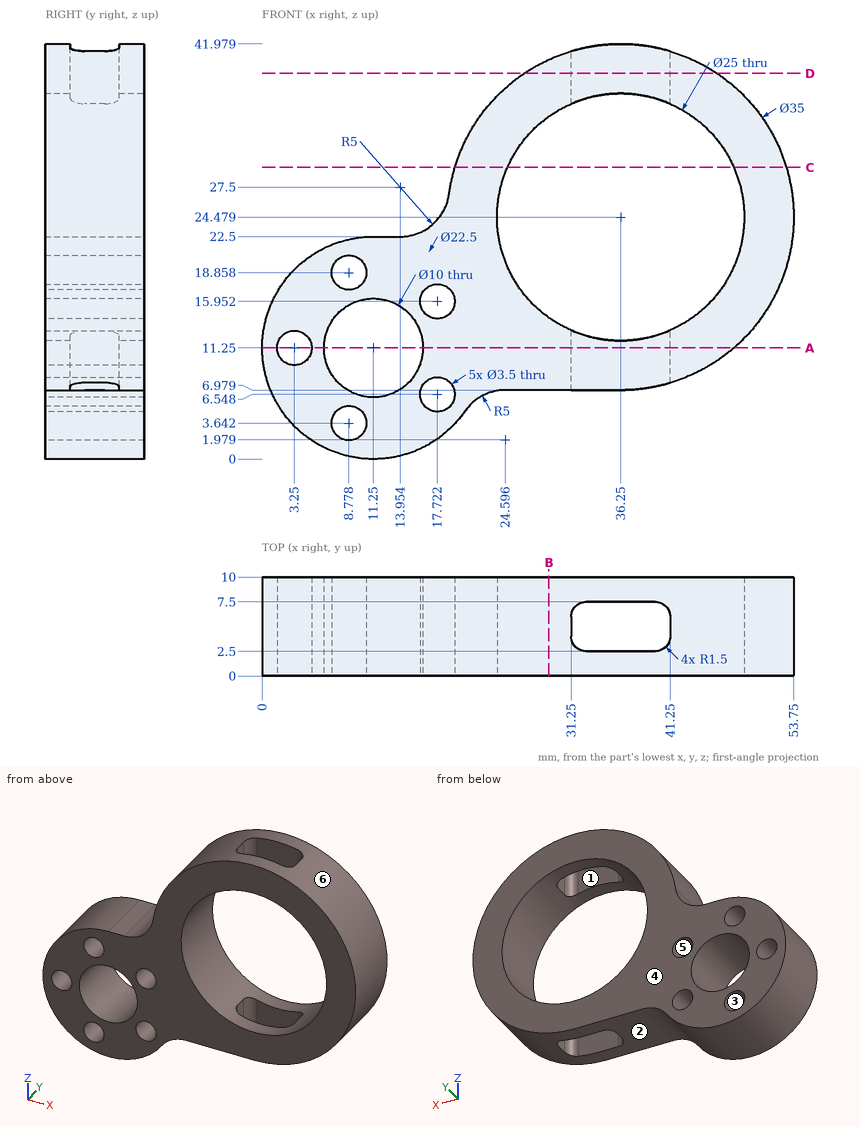
Drawing for the job (mm, zero at the part's lowest x, y, z). A direction names the side the tool comes from. Coordinates: 2 decimals unless noted, no trailing zeros. Order: outer loops, then holes, each group sorted by start corner. A loop starts at its lowest first (then second) coordinate and runs counter-clockwise, first axis right, second up. Notation, with made-up numbers: (-32, -10) - (9, -10) arc R19 ccw to (9, 18) - close; hole circle Ø5 at (-9.5, -0.75). An arc over 180 degrees is marked (long way). Use a Markdown table: item, result. Add a question column.
(1) Which spindle directions (+Z, -Z, +X, -X, +Y, -Y) get a long thin tool onto all of the face, cutting with end or side? Do the marked faces 1, 2 and 3. Say none if no direction does.
(2) Saw through at A-A (z = 11.25). Give the cut face in (x, y), then the cut area to 3 significant figures.
(3) Saw through at C-C (z = 29.5). Give the cut face in (x, y) (1 decimal).
(4) Drill centre lines: line 1 along Z through (x, y) = (11, 7); line 2 along X through (y, z) = (8.25, 34.5) (1 decimal); line 3 along X through (y, z) = (7, 36.5). Where is each one in solid material? Low to high. Write a range as [from, to].
(5) Saw through at D-D (z = 39). Give the cut face in (x, y).
(6) Saw through at B-B (x = 29). Give the cut face in (y, z).
(7) Pull direction X, two halves, no side cores. Call the marked faces 4, 5 and 6: +X half, -X half, draft (parallel to the pull), parting line (faces both ways), or undercut.
(8) Flat gauge pins, fed straight in: pin 1 (4.5 mm diameter, centred on x = 8.78, z = 18.86, fed in from -Y); pin 2 (1 mm diameter, centred on x = 9, y = 6, fed in from +Z); pin 3 (1.6 mm diameter, centred on y = 5, z = 39, fed in from -X); pin 4 (2 mm diameter, centred on y = 4.5, z = 38.5, fed in from +X). Where does each tip first touch, or does it go through?
Solved:
| question | item | result |
|---|---|---|
| 1 | face 1 | +Z, -Z |
| 1 | face 2 | -Z, +X, +Y, -Y |
| 1 | face 3 | +Y, -Y |
| 2 | outline | (0, 0) - (1.5, 0) - (1.5, 10) - (0, 10) - close; (5, 0) - (6.25, 0) - (6.25, 10) - (5, 10) - close; (16.25, 0) - (47.71, 0) - (47.71, 10) - (16.25, 10) - close; hole (31.25, 4) arc R1.5 ccw to (32.75, 2.5) - (39.75, 2.5) arc R1.5 ccw to (41.25, 4) - (41.25, 6) arc R1.5 ccw to (39.75, 7.5) - (32.75, 7.5) arc R1.5 ccw to (31.25, 6) - close |
| 2 | area | 294 mm² |
| 3 | outline | (19.5, 0) - (24.8, 0) - (24.8, 10) - (19.5, 10) - close; (47.7, 0) - (53, 0) - (53, 10) - (47.7, 10) - close |
| 4 | line 1 | z = [0, 6.26], [16.24, 22.5] |
| 4 | line 2 | x = [21.9, 28.8], [43.7, 50.6] |
| 4 | line 3 | x = [23.53, 31.63], [40.87, 48.97] |
| 5 | outline | (26.48, 0) - (46.02, 0) - (46.02, 10) - (26.48, 10) - close; hole (31.25, 4) arc R1.5 ccw to (32.75, 2.5) - (39.75, 2.5) arc R1.5 ccw to (41.25, 4) - (41.25, 6) arc R1.5 ccw to (39.75, 7.5) - (32.75, 7.5) arc R1.5 ccw to (31.25, 6) - close |
| 6 | outline | (0, 6.98) - (10, 6.98) - (10, 14.3) - (0, 14.3) - close; (0, 34.66) - (10, 34.66) - (10, 40.41) - (0, 40.41) - close |
| 7 | face 4 | draft |
| 7 | face 5 | undercut |
| 7 | face 6 | parting line |
| 8 | pin 1 | stops at y = 0 |
| 8 | pin 2 | stops at z = 22.36 |
| 8 | pin 3 | stops at x = 25.39 |
| 8 | pin 4 | stops at x = 47.94 |
